from build123d import *

# Parameters (mm, degrees)
SKETCH1_R           = 15
BOSS_EXTRUDE1_DEPTH = 10


with BuildPart() as part:
    # Sketch1 → Boss-Extrude1 (new body)
    with BuildSketch(Plane.XY):
        with BuildLine():
            Line((22.913573162, 19.378039256), (19.356826052, 15.821292146))
            ThreePointArc((19.356826052, 15.821292146), (23.096988313, 9.567085809), (24.874685928, 2.5))
            Line((24.874685928, 2.5), (29.9, 2.5))
            Line((29.9, 2.5), (29.9, -2.5))
            Line((29.9, -2.5), (24.874685928, -2.5))
            ThreePointArc((24.874685928, -2.5), (23.096988313, -9.567085809), (19.356826052, -15.821292146))
            Line((19.356826052, -15.821292146), (22.913573162, -19.378039256))
            Line((22.913573162, -19.378039256), (19.378039256, -22.913573162))
            Line((19.378039256, -22.913573162), (15.821292146, -19.356826052))
            ThreePointArc((15.821292146, -19.356826052), (9.567085809, -23.096988313), (2.5, -24.874685928))
            Line((2.5, -24.874685928), (2.5, -29.9))
            Line((2.5, -29.9), (-2.5, -29.9))
            Line((-2.5, -29.9), (-2.5, -24.874685928))
            ThreePointArc((-2.5, -24.874685928), (-9.567085809, -23.096988313), (-15.821292146, -19.356826052))
            Line((-15.821292146, -19.356826052), (-19.378039256, -22.913573162))
            Line((-19.378039256, -22.913573162), (-22.913573162, -19.378039256))
            Line((-22.913573162, -19.378039256), (-19.356826052, -15.821292146))
            ThreePointArc((-19.356826052, -15.821292146), (-23.096988313, -9.567085809), (-24.874685928, -2.5))
            Line((-24.874685928, -2.5), (-29.9, -2.5))
            Line((-29.9, -2.5), (-29.9, 2.5))
            Line((-29.9, 2.5), (-24.874685928, 2.5))
            ThreePointArc((-24.874685928, 2.5), (-23.096988313, 9.567085809), (-19.356826052, 15.821292146))
            Line((-19.356826052, 15.821292146), (-22.913573162, 19.378039256))
            Line((-22.913573162, 19.378039256), (-19.378039256, 22.913573162))
            Line((-19.378039256, 22.913573162), (-15.821292146, 19.356826052))
            ThreePointArc((-15.821292146, 19.356826052), (-9.567085809, 23.096988313), (-2.5, 24.874685928))
            Line((-2.5, 24.874685928), (-2.5, 29.9))
            Line((-2.5, 29.9), (2.5, 29.9))
            Line((2.5, 29.9), (2.5, 24.874685928))
            ThreePointArc((2.5, 24.874685928), (9.567085809, 23.096988313), (15.821292146, 19.356826052))
            Line((15.821292146, 19.356826052), (19.378039256, 22.913573162))
            Line((19.378039256, 22.913573162), (22.913573162, 19.378039256))
        make_face()
        Circle(SKETCH1_R, mode=Mode.SUBTRACT)
    extrude(amount=BOSS_EXTRUDE1_DEPTH)


solid = part.part
For this review, take the finished solid that the model builds, in its own axes (mm). A direction names the side the tool comes from. Coordinates: 2 decimals unless noted, no trailing zeros. Loops run counter-clockwise (first coordinate to the right, second up) from the corner with the lowest first, then second, coordinate; pieces in that order, holes last. Notation, with made-up numbers: (-34, 28.25) - (9, 28.25) arc R25 cw to (9, 45.25) - close; hole circle Ø10 at (37, 62.25). An arc over 180 degrees is marked (long way). Use a Markdown table: item, result. Add a question column.
Item 1: We need section A-A (x = 0). Give the boundary of the cut face in (y, z).
Item 2: Tool access review of faces 4 (the face through (17.625, -21.16, 4.93)), 5 (the face through (-9.66, 23.06, 4.93)), 6 (the face through (23.06, 9.66, 4.93)): name each direction out of +Z, -Z, +X, -X, +Y, -Y from which nothing blocks a thin tool from reaching the whole face with its end or side.
Item 3: Mouldability with a two-part tool opening along X and no side actions: class faces 1 (the face through (-14.985, 0.66, 4.93)), 2 (the face through (29.9, 0, 5)), 3 (the face through (-29.9, 0, 5)) as pulls with the +X half, pulls with the -X half, needs draft (parallel to the pull), parting line crosses it, or undercut.
Item 4: For line 1 (Y direction, x = 0, z = 8.75); line 2 (X direction, y = -27, z = 6); line 3 (Y direction, x = -11, z = 3.25), list the stretches that pass through material, from the lowest coordinate up.
Item 5: Insertion check: pin 1 Ø1 at (y, z) = (10.5, 9) entering from +X; pin 2 Ø5.5 at (y, z) = (28.5, 6) entering from +X; pin 3 Ø5.5 at (x, z) = (28.5, 6) entering from -Y. Each pin has a flat end and moves straight along its axis. Give the tip position at first contact, or say it passes through.
Item 6: We need section D-D (y = -24). Give the boundary of the cut face in (x, z).
Results list:
| question | item | result |
|---|---|---|
| 1 | outline | (-29.9, 0) - (-15, 0) - (-15, 10) - (-29.9, 10) - close; (15, 0) - (29.9, 0) - (29.9, 10) - (15, 10) - close |
| 2 | face 4 | +Z, -Z, -Y |
| 2 | face 5 | +Z, -Z, +Y |
| 2 | face 6 | +Z, -Z, +X |
| 3 | face 1 | undercut |
| 3 | face 2 | pulls with the +X half |
| 3 | face 3 | pulls with the -X half |
| 4 | line 1 | y = -29.9 to -15, 15 to 29.9 |
| 4 | line 2 | x = -2.5 to 2.5 |
| 4 | line 3 | y = -22.45 to -10.2, 10.2 to 22.45 |
| 5 | pin 1 | stops at x = 22.91 |
| 5 | pin 2 | stops at x = 2.5 |
| 5 | pin 3 | stops at y = -2.5 |
| 6 | outline | (-7, 0) - (7, 0) - (7, 10) - (-7, 10) - close |
